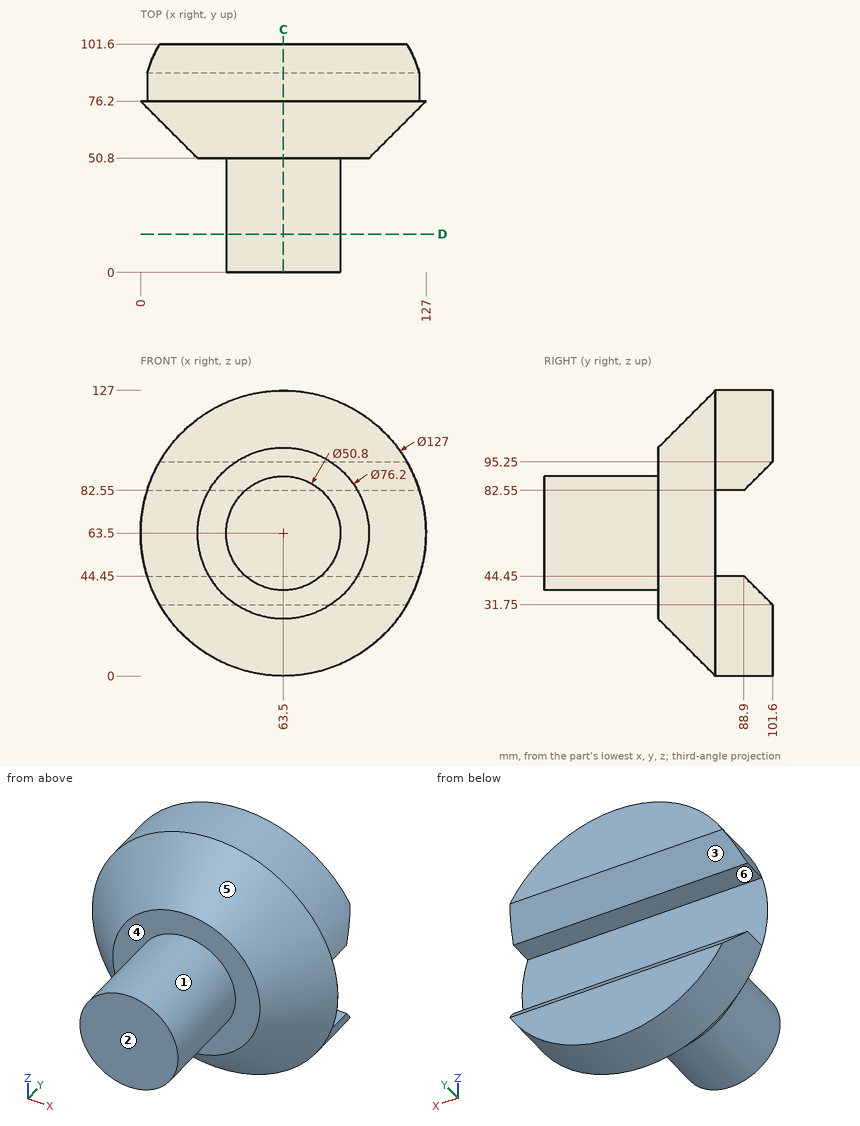
Design review of the part shown in the three views and the two pictorial views. Dimensions are in mm from the part's minimum x, y and z. A direction names the side the tool comes from. Give positions to 0.01 mm unless a question says otherwise; leave off trailing zeros. Write each loop counter-clockwise with the first axis right and the second up, starting at its lowest first coordinate (ties: lowest second). Pieces come first, ordered by that corner, then holes. Notation, with made-up numbers: M 72.25,-28.75 L 127.25,-28.75 A29 ccw 127.25,6.25 Z; hole C 70,-17.5 d4. An arc over 180 degrees is marked long. One line per question, with ' | ' between items. Start each with the question number.
Item 1: Draft analysis for pull direction Z (two halves, no side actions). For the marked faces 4, 5 and 6, state which applies: released by +Z, released by -Z, zero draft, split by the parting line, or undercut.
Item 2: For the marked faces 1, 2 and 3, list the 3-axis set-ups (+Z, -Z, +X, -X, +Y, -Y) from which the entire face can be reached by the end or side of a thin tool; tool diameter is ignored.
Item 3: For pin 1 (10 mm diameter, centred on x = 59.5, y = 40, fed in from +Z); pin 2 (10 mm diameter, centred on x = 24.5, y = 54, fed in from -Z); pin 3 (10 mm diameter, centred on x = 19.5, z = 72, fed in from +Y), all flat-tipped, find the tip position at first contact; note any pin that passes through.
Item 4: We need section D-D on y = 17. Write out the cut boundary in (x, z).
Item 5: We need section C-C on x = 63.5. Write out the cut boundary in (y, z), plus the area to 3 significant figures.
Item 6: Wall thickness on line 1 (Y direction, x = 72, z = 81); line 2 (Y direction, x = 41.5, z = 79.5); line 3 (Z direction, x = 41, y = 77): over which ranges is each line inside the solid? List them lowest first. Write a range as from..to.
Results found:
1) face 4: zero draft | face 5: split by the parting line | face 6: undercut
2) face 1: -Y | face 2: +Z, -Z, +X, -X, -Y | face 3: +X, -X, +Y
3) pin 1: stops at z = 88.9 | pin 2: stops at z = 36 | pin 3: stops at y = 76.2
4) outline: C 63.5,63.5 d50.8
5) outline: M 0,38.1 L 50.8,38.1 L 50.8,25.4 L 76.2,0 L 101.6,0 L 101.6,31.75 L 88.9,44.45 L 76.2,44.45 L 76.2,82.55 L 88.9,82.55 L 101.6,95.25 L 101.6,127 L 76.2,127 L 50.8,101.6 L 50.8,88.9 L 0,88.9 Z | area: 7,260 mm2
6) line 1: y = 0..76.2 | line 2: y = 50.8..76.2 | line 3: z = 4.12..44.45, 82.55..122.88
